```python
from build123d import *

# Parameters (mm, degrees)
SKETCH1_W           = 300
SKETCH1_H           = 900
BOSS_EXTRUDE1_DEPTH = 600
SKETCH4_W           = 150.6
SKETCH4_H           = 150
BOSS_EXTRUDE3_DEPTH = 120
SKETCH6_W           = 150.6
SKETCH6_H           = 150
BOSS_EXTRUDE4_DEPTH = 120
FILLET1_R           = 10
FILLET2_R           = 10
FILLET3_R           = 10
FILLET5_R           = 10
FILLET6_R           = 10
SKETCH8_W           = 260
SKETCH8_H           = 560
CUT_EXTRUDE1_DEPTH  = 1161.344776349
SKETCH7_W           = 100.6
SKETCH7_H           = 100
CUT_EXTRUDE2_DEPTH  = 1209.966500777


with BuildPart() as part:
    # Sketch1 → Boss-Extrude1 (new body)
    with BuildSketch(Plane.XY):
        with Locations((150, -450)):
            Rectangle(SKETCH1_W, SKETCH1_H)
    extrude(amount=-BOSS_EXTRUDE1_DEPTH)

    # Sketch4 → Boss-Extrude3 (add)
    with BuildSketch(Plane(origin=(300, 0, 0), x_dir=(0, 0, -1), z_dir=(1, 0, 0))):
        with Locations((300, -175)):
            Rectangle(SKETCH4_W, SKETCH4_H)
    extrude(amount=BOSS_EXTRUDE3_DEPTH)

    # Sketch6 → Boss-Extrude4 (add)
    with BuildSketch(Plane.ZY):
        with Locations((-300, -175)):
            Rectangle(SKETCH6_W, SKETCH6_H)
    extrude(amount=BOSS_EXTRUDE4_DEPTH)

    # Fillet1
    fillet1_edges = [part.edges().sort_by_distance(p)[0] for p in [
        (300, -450, -600),
        (0, -450, -600),
        (0, 0, -300),
    ]]
    fillet(fillet1_edges, radius=FILLET1_R)

    # Fillet2
    fillet2_edges = [part.edges().sort_by_distance(p)[0] for p in [
        (0, -175, -224.7),
        (-60, -250, -224.7),
        (0, -100, -300),
        (-60, -100, -224.7),
        (0, -175, -375.3),
        (-60, -100, -375.3),
        (0, -250, -300),
        (-60, -250, -375.3),
        (-120, -175, -224.7),
        (-120, -100, -300),
        (-120, -175, -375.3),
        (-120, -250, -300),
    ]]
    fillet(fillet2_edges, radius=FILLET2_R)

    # Fillet3
    fillet3_edges = [part.edges().sort_by_distance(p)[0] for p in [
        (300, -175, -375.3),
        (360, -250, -375.3),
        (300, -100, -300),
        (360, -100, -375.3),
        (300, -175, -224.7),
        (360, -100, -224.7),
        (300, -250, -300),
        (360, -250, -224.7),
        (420, -175, -375.3),
        (420, -100, -300),
        (420, -175, -224.7),
        (420, -250, -300),
    ]]
    fillet(fillet3_edges, radius=FILLET3_R)

    # Fillet5
    # the kernel refuses this fillet: 10 mm, written as the material it takes off along each edge
    with BuildSketch(Plane(origin=(10, -10, -590), x_dir=(0, 0, -1), z_dir=(0, 1, 0))) as fillet5_piece_1_section:
        Polygon((0, 0), (FILLET5_R, 0), (FILLET5_R, FILLET5_R), (0, FILLET5_R), align=None)
    fillet5_piece_1 = extrude(amount=FILLET5_R, mode=Mode.PRIVATE)
    fillet5_piece_1 = fillet5_piece_1 - Plane(origin=(10, -10, -590), x_dir=(0.7071067811865475, 0, 0.7071067811865475), z_dir=(0, 1, 0)) * Sphere(FILLET5_R, mode=Mode.PRIVATE)
    add(fillet5_piece_1, mode=Mode.SUBTRACT)
    with BuildSketch(Plane(origin=(300, 0, 25), x_dir=(0, -1, 0), z_dir=(0, 0, -1))) as fillet5_piece_2:
        with BuildLine():
            CenterArc((FILLET5_R, FILLET5_R), FILLET5_R, 180, 90)
            Line((0, FILLET5_R), (0, 0))
            Line((0, 0), (FILLET5_R, 0))
        make_face()
    extrude(amount=615, mode=Mode.SUBTRACT)
    with BuildSketch(Plane(origin=(10, 0, -600), x_dir=(0, 0, 1), z_dir=(1, 0, 0))) as fillet5_piece_3:
        with BuildLine():
            CenterArc((FILLET5_R, FILLET5_R), FILLET5_R, 180, 90)
            Line((0, FILLET5_R), (0, 0))
            Line((0, 0), (FILLET5_R, 0))
        make_face()
    extrude(amount=280, mode=Mode.SUBTRACT)
    with BuildSketch(Plane(origin=(290, 0, -590), x_dir=(1, 0, 0), z_dir=(0, 0, 1))) as fillet5_piece_4:
        with BuildLine():
            CenterArc((10 - FILLET5_R, -FILLET5_R), FILLET5_R, 0, 90)
            Line((10, -FILLET5_R), (10, 0))
            Line((10, 0), (10 - FILLET5_R, 0))
        make_face()
    revolve(axis=Axis((290, 0, -590), (0, 1, 0)), revolution_arc=90, mode=Mode.SUBTRACT)

    # Fillet6
    fillet6_edges = [part.edges().sort_by_distance(p)[0] for p in [
        (150, 0, 0),
        (297.071067812, -2.928932188, 0),
        (0, -455, 0),
        (2.928932188, -2.928932188, 0),
        (300, -455, 0),
    ]]
    fillet(fillet6_edges, radius=FILLET6_R)

    # Sketch8 → Cut-Extrude1 (cut, through all)
    with BuildSketch(Plane.XZ.offset(900)):
        with Locations((150, -300)):
            Rectangle(SKETCH8_W, SKETCH8_H)
    extrude(amount=-CUT_EXTRUDE1_DEPTH, mode=Mode.SUBTRACT)

    # Sketch7 → Cut-Extrude2 (cut, through all)
    with BuildSketch(Plane.ZY.offset(120)):
        with Locations((-300, -175)):
            Rectangle(SKETCH7_W, SKETCH7_H)
    extrude(amount=-CUT_EXTRUDE2_DEPTH, mode=Mode.SUBTRACT)


solid = part.part
```
For this review, take the finished solid that the model builds, in its own axes (mm). A direction names the side the tool comes from. Coordinates: 2 decimals unless noted, no trailing zeros. Order: outer loops, then holes, each group sorted by start corner. A loop starts at its lowest first (then second) coordinate and runs counter-clockwise, first axis right, second up. Notation, with made-up numbers: (7, 37.25) -> (56, 37.25) arc R21 ccw to (56, 72.25) -> close; hole circle Ø3 at (33.5, -30.5). An arc over 180 degrees is marked (long way). Use CSV: the item, a comma, the result in double quotes. Start each with the question number.
Item 1: Draft analysis for pull direction Z (two halves, no side actions). For faces 1 (the face through (-59, -250, -301)), 2 (the face through (349, -176, -350.3)), 3 (the face through (359, -176, -224.7)), state which applies: pulls with the +Z half, pulls with the -Z half, needs draft (parallel to the pull), parting line crosses it, or undercut.
Item 2: We need section D-D, the plane y = -652. Give the boundary of the cut face in (x, z).
Item 3: We need section A-A, the plane z = -315.5. Give the number of separate pieces and of enclosed holes in the cut face, then the cut area to 3 significant figures.
Item 4: Wall thickness on probe 1 along Z at (x, y) = (263, -248); probe 2 along X at (y, z) = (-45.5, -314); probe 3 along Y at (x, z) = (-14, -274): over which ranges is each line inside the solid? List them lowest first.
Item 5: We need section B-B, the plane x = 256. Give the boundary of the cut face in (y, z).
Item 6: We need section C-C, the plane z = -201.5. Give the boundary of the cut face in (x, y).
Item 7: Insertion check: pin 1 (1.5 mm diameter, centred on y = -107, z = -291.5, fed in from -X); pin 2 (1 mm diameter, centred on y = -131.5, z = -432, fed in from +X). Each pin has a flat end and moves straight along its axis. Give the tip position at first contact, or say it passes through.
Item 8: For faces 4 (the face through (280, -456, -304)), 5 (the face through (-59, -100, -301)), 6 (the face through (359, -176, -375.3)), 7 (the face through (359, -250, -299)), 8 (the face through (-51, -225, -301)), list the 3-axis set-ups (+Z, -Z, +X, -X, +Y, -Y) from which the entire face can be reached by the end or side of a thin tool; tool diameter is ignored.
Derived:
1,face 1,"needs draft"
1,face 2,"undercut"
1,face 3,"pulls with the +Z half"
2,outline,"(0, -590) arc R10 ccw to (10, -600) -> (290, -600) arc R10 ccw to (300, -590) -> (300, -10) arc R10 ccw to (290, 0) -> (10, 0) arc R10 ccw to (0, -10) -> close; hole (20, -580) -> (280, -580) -> (280, -20) -> (20, -20) -> close"
3,separate pieces,"4"
3,enclosed holes,"0"
3,area,"44,000 mm^2"
4,probe 1,"z = -600 to -580, -20 to 0"
4,probe 2,"x = 0 to 20, 280 to 300"
4,probe 3,"y = -250 to -225, -125 to -100"
5,outline,"(-900, -600) -> (-10, -600) arc R10 ccw to (0, -590) -> (0, -580) -> (-900, -580) -> close; (-900, -20) -> (0, -20) -> (0, -10) arc R10 ccw to (-10, 0) -> (-900, 0) -> close"
6,outline,"(0, -900) -> (20, -900) -> (20, 0) -> (10, 0) arc R10 ccw to (0, -10) -> close; (280, -900) -> (300, -900) -> (300, -10) arc R10 ccw to (290, 0) -> (280, 0) -> close"
7,pin 1,"stops at x = -119.74"
7,pin 2,"stops at x = 300"
8,face 4,"+Y, -Y"
8,face 5,"+Z, -Z, -X, +Y"
8,face 6,"-Z, +X, +Y, -Y"
8,face 7,"+Z, -Z, +X, -Y"
8,face 8,"+X, -X"
